Autodesk Inventor part; units mm, degrees
ref_plane "YZ Plane" through (0, 0, 0) normal (1, 0, 0) x (0, 1, 0)
ref_plane "XZ Plane" through (0, 0, 0) normal (0, 1, 0) x (-1, 0, 0)
ref_plane "XY Plane" through (0, 0, 0) normal (0, 0, 1) x (1, 0, 0)
sketch "Sketch1" plane through (0, 0, 0) normal (0, 0, 1) x (1, 0, 0)
  circle A0 centre (0, 0) radius 2.7432
  dimension "d0" = 5.4864
extrude "Extrusion1" add sketch "Sketch1" against normal blind 9.525
sketch "Sketch2" plane through (0, 0, -9.525) normal (0, 0, -1) x (-1, 0, 0)
  circle A0 centre (0, 0) radius 2.7432
  circle A1 centre (0, 0) radius 1.778
  dimension "d3" = 3.556
extrude "Extrusion2" add sketch "Sketch2" along normal blind 9.525 contours A1
thread "Thread1"
sketch "Sketch3" plane through (0, 0, 0) normal (0, 0, 1) x (1, 0, 0)
  circle A0 centre (0, 0) radius 2.7432
  line L0 (-0.3969, 2.7143) -> (-0.3969, -2.7143)
  line L1 (0.3969, -2.7143) -> (0.3969, 2.7143)
  dimension "d8" = 0.7937
  dimension "d9" = 0.3969
extrude "Extrusion3" cut sketch "Sketch3" against normal blind 1.1906 contours L1 A0 L0
equation "\"d9\" = 0.5 * d8"
properties part number "Set_Screw" material "Steel, Mild"
Source: CAD feature listing. Evaluate the final solid. Frame: model axes, mm. A direction names the side the tool comes from. Coordinates: 2 decimals unless noted, no trailing zeros. Order: outer loops, then holes, each group sorted by start corner. A loop starts at its lowest first (then second) coordinate and runs counter-clockwise, first axis right, second up.
Item 1: Cut plane D-D (y = -1). Return loops of the section in (x, z) (3 decimals), plus the area to 3 significant figures.
Output values:
outline: (-2.554, -9.525) - (-1.47, -9.525) - (-1.47, -19.05) - (1.47, -19.05) - (1.47, -9.525) - (2.554, -9.525) - (2.554, 0) - (0.397, 0) - (0.397, -1.191) - (-0.397, -1.191) - (-0.397, 0) - (-2.554, 0) - close
area: 75.7 mm2
Item 2: Cut plane C-C (z = -9). Return loops of the section in (x, y).
Output values:
outline: circle Ø5.49 at (0, 0)
Item 3: Material intervals for line 1 (Z direction, x = -1.25, y = 1.4) (3 decimals); line 2 (X direction, y = -0.4, z = -6.5); line 3 (Z direction, x = 0.3, y = -2.5) (3 decimals), sorted ascending.
Output values:
line 1: z = -9.525 to 0
line 2: x = -2.71 to 2.71
line 3: z = -9.525 to -1.191
Item 4: Cut plane B-B (x = 0). Return loops of the section in (y, z) (3 decimals), plus the area to 3 significant figures.
Output values:
outline: (-2.743, -9.525) - (-1.778, -9.525) - (-1.778, -19.05) - (1.778, -19.05) - (1.778, -9.525) - (2.743, -9.525) - (2.743, -1.191) - (-2.743, -1.191) - close
area: 79.6 mm2
Item 5: Set-up query: faces 4 (the face through (-0.397, 0, -1)), 5 (the face through (0.385, 1.736, -14.221)), 6 (the face through (-1, 0, 0)). Return all of +Z, -Z, +X, -X, +Y, -Y with unobstructed straight access to the full face (end or side cutting, diameter ignored); none if empty.
Output values:
face 4: +Z, +Y, -Y
face 5: -Z
face 6: +Z, +X, -X, +Y, -Y
Item 6: Pull-direction query (X, two-part tool) for faces 1 (the face through (-0.59, -2.68, -4.7)), 2 (the face through (0.397, 0, -1)), 3 (the face through (1, 0, 0)); classes: pulls with the +X half, pulls with the -X half, needs draft (parallel to the pull), parting line crosses it, or undercut.
Output values:
face 1: parting line crosses it
face 2: undercut
face 3: needs draft
Item 7: First-contact query: P1, Ø1.5, axis at x = 1, y = 2, coming from the -Z side; P2, Ø1.3, axis at y = -1, z = -0.5, coming from the +X side; P3, Ø0.6, axis at x = 0, y = 1, coming from the +Z side. Flat tips, straight axial feed; report the tip coordinate or a pass-through.
Output values:
P1: stops at z = -19.05
P2: stops at x = 2.72
P3: stops at z = -1.19
Item 8: Cut plane A-A (y = 0). Return loops of the section in (x, z) (3 decimals).
Output values:
outline: (-2.743, -9.525) - (-1.778, -9.525) - (-1.778, -19.05) - (1.778, -19.05) - (1.778, -9.525) - (2.743, -9.525) - (2.743, 0) - (0.397, 0) - (0.397, -1.191) - (-0.397, -1.191) - (-0.397, 0) - (-2.743, 0) - close
